from build123d import *

# Parameters (mm, degrees)
BOSS_EXTRUDE1_DEPTH = 4
SKETCH2_R           = 2.4
CUT_EXTRUDE1_DEPTH  = 12.510864433
SKETCH3_R           = 3.1
CUT_EXTRUDE2_DEPTH  = 1


with BuildPart() as part:
    # Sketch1 → Boss-Extrude1 (new, symmetric)
    with BuildSketch(Plane(origin=(0, 0, 0), x_dir=(1, 0, 0), z_dir=(0, 1, 0))):
        with BuildLine():
            Line((-4, 3.5), (4, 3.5))
            ThreePointArc((4, 3.5), (7.5, 0), (4, -3.5))
            Line((4, -3.5), (-4, -3.5))
            ThreePointArc((-4, -3.5), (-7.5, 0), (-4, 3.5))
        make_face()
    extrude(amount=BOSS_EXTRUDE1_DEPTH, both=True)

    # Sketch2 → Cut-Extrude1 (cut, through all)
    with BuildSketch(Plane(origin=(0, 4, 0), x_dir=(1, 0, 0), z_dir=(0, 1, 0))):
        with Locations(Location((4, 0, 0), (0, 0, 270))):
            Circle(SKETCH2_R)
        with BuildLine():
            Line((-4.84, -2.177705214), (-4.84, -1.24))
            ThreePointArc((-4.84, -1.24), (-4.957157288, -0.957157288), (-5.24, -0.84))
            Line((-5.24, -0.84), (-6.177705214, -0.84))
            ThreePointArc((-6.177705214, -0.84), (-6.235940121, -0.821293884), (-6.27238805, -0.772173913))
            ThreePointArc((-6.27238805, -0.772173913), (-6.4, 0), (-6.27238805, 0.772173913))
            ThreePointArc((-6.27238805, 0.772173913), (-6.235940121, 0.821293884), (-6.177705214, 0.84))
            Line((-6.177705214, 0.84), (-5.24, 0.84))
            ThreePointArc((-5.24, 0.84), (-4.957157288, 0.957157288), (-4.84, 1.24))
            Line((-4.84, 1.24), (-4.84, 2.177705214))
            ThreePointArc((-4.84, 2.177705214), (-4.821293884, 2.235940121), (-4.772173913, 2.27238805))
            ThreePointArc((-4.772173913, 2.27238805), (-4, 2.4), (-3.227826087, 2.27238805))
            ThreePointArc((-3.227826087, 2.27238805), (-3.178706116, 2.235940121), (-3.16, 2.177705214))
            Line((-3.16, 2.177705214), (-3.16, 1.24))
            ThreePointArc((-3.16, 1.24), (-3.042842712, 0.957157288), (-2.76, 0.84))
            Line((-2.76, 0.84), (-1.822294786, 0.84))
            Line((-1.822294786, 0.84), (-0.602294892, 0.84))
            ThreePointArc((-0.602294892, 0.84), (-0.767197546, 1.341263694), (-1.005585937, 1.812038747))
            ThreePointArc((-1.005585937, 1.812038747), (-1.042652048, 2.255086643), (-0.7121875, 2.552506408))
            ThreePointArc((-0.7121875, 2.552506408), (0, 2.65), (0.7121875, 2.552506408))
            ThreePointArc((0.7121875, 2.552506408), (1.042652048, 2.255086643), (1.005585937, 1.812038747))
            ThreePointArc((1.005585937, 1.812038747), (0.5, 0), (1.005585938, -1.812038747))
            ThreePointArc((1.005585938, -1.812038747), (1.042652048, -2.255086643), (0.7121875, -2.552506408))
            ThreePointArc((0.7121875, -2.552506408), (0, -2.65), (-0.7121875, -2.552506408))
            ThreePointArc((-0.7121875, -2.552506408), (-1.042652048, -2.255086643), (-1.005585937, -1.812038747))
            ThreePointArc((-1.005585937, -1.812038747), (-0.767197546, -1.341263694), (-0.602294892, -0.84))
            Line((-0.602294892, -0.84), (-1.822294786, -0.84))
            Line((-1.822294786, -0.84), (-2.76, -0.84))
            ThreePointArc((-2.76, -0.84), (-3.042842712, -0.957157288), (-3.16, -1.24))
            Line((-3.16, -1.24), (-3.16, -2.177705214))
            ThreePointArc((-3.16, -2.177705214), (-3.178706116, -2.235940121), (-3.227826087, -2.27238805))
            ThreePointArc((-3.227826087, -2.27238805), (-4, -2.4), (-4.772173913, -2.27238805))
            ThreePointArc((-4.772173913, -2.27238805), (-4.821293884, -2.235940121), (-4.84, -2.177705214))
        make_face()
    extrude(amount=-CUT_EXTRUDE1_DEPTH, mode=Mode.SUBTRACT)

    # Sketch3 → Cut-Extrude2 (cut)
    with BuildSketch(Plane(origin=(0, 4, 0), x_dir=(1, 0, 0), z_dir=(0, 1, 0))):
        with Locations(Location((4, 0, 0), (0, 0, 270))):
            Circle(SKETCH3_R)
    cut_extrude2 = extrude(amount=-CUT_EXTRUDE2_DEPTH, mode=Mode.SUBTRACT)

    # Mirror1: Cut-Extrude2 across plane
    add(cut_extrude2.mirror(Plane.ZX), mode=Mode.SUBTRACT)


solid = part.part
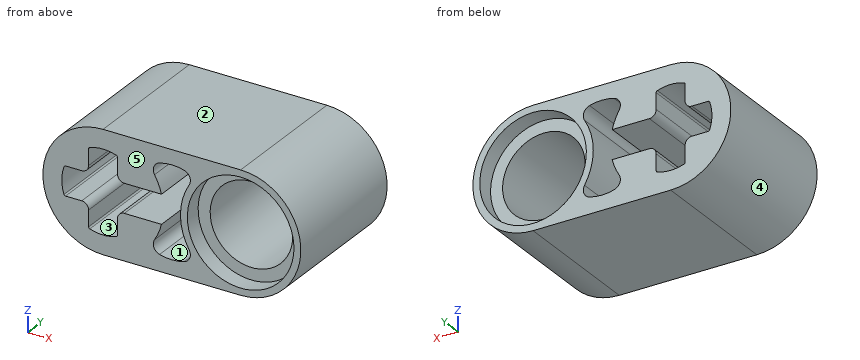
Could you check a few things on this model? Use its own coordinates, in mm. Face numbers are marked on the shaded views. A direction names the side the tool comes from. Round coordinates to 2 decimals unless told otherwise and drop trailing zeros. Loops run counter-clockwise (first coordinate to the right, second up) from the corner with the lowest first, then second, coordinate; pieces in that order, holes last. Notation, with made-up numbers: (72.25, -14.5) - (82.25, -14.5) arc R20 ccw to (82.25, -4.5) - close; hole circle Ø7 at (64.5, 34.25). An arc over 180 degrees is marked (long way). Write item = value, one per line.
1) Imagine slicing it at B-B (x = 5.5). Please give me the cut outline in (y, z), and give its area (3 significant figures).
Computed:
outline = (-4, -3.16) - (4, -3.16) - (4, -2.71) - (3, -2.71) - (3, -1.87) - (-3, -1.87) - (-3, -2.71) - (-4, -2.71) - close; (-4, 2.71) - (-3, 2.71) - (-3, 1.87) - (3, 1.87) - (3, 2.71) - (4, 2.71) - (4, 3.16) - (-4, 3.16) - close
area = 17.3 mm2
2) On a 3-axis mill with a long thin cutter (end or side, diameter ignored), from which of +Z, -Z, +X, -X, +Y, -Y can I reach the whole of each face in a straight line? I mean the marked faces 1 and 2. Say none if no direction works.
Computed:
face_1 = +Y, -Y
face_2 = +Z, +X, -X, +Y, -Y
3) Imagine slicing it at A-A (z = -2). Please give me the cut outline in (x, y), and give its area (3 significant figures).
Computed:
outline = (-6.87, -4) - (-4.84, -4) - (-4.84, 4) - (-6.87, 4) - close; (-3.16, -4) - (-1.07, -4) - (-1.07, 4) - (-3.16, 4) - close; (1.07, -4) - (1.63, -4) - (1.63, -3) - (2.67, -3) - (2.67, 3) - (1.63, 3) - (1.63, 4) - (1.07, 4) - close; (5.33, -3) - (6.37, -3) - (6.37, -4) - (6.87, -4) - (6.87, 4) - (6.37, 4) - (6.37, 3) - (5.33, 3) - close
area = 54.0 mm2
4) If we mould it in two halves opening along Z, with no side actions, what happens to the marked faces 3, 4 and 5? For each: pulls with the +Z half, pulls with the -Z half, needs draft (parallel to the pull), parting line crosses it, or undercut.
Computed:
face_3 = undercut
face_4 = parting line crosses it
face_5 = needs draft
5) I need wall thicknesses on line 1 along Y through (x, z) = (6.75, 0.25); line 2 along Z through (x, y) = (-2.25, 1.25); line 3 along Z through (x, y) = (-1, 0.5). Which ranges of each line are inside material? Lowest first, please. Write a range as from..to.
Computed:
line_1 = -3..3
line_2 = -3.5..-0.84, 0.84..3.5
line_3 = -3.5..-2.34, -1.8..-0.84, 0.84..1.8, 2.34..3.5
6) I'm going to push flat-ended pins straight in: P1, Ø0.5, axis at x = -5.5, y = 0.5, coming from the -Z side; P2, Ø1, axis at y = 1.5, z = 1.5, coming from the -X side; P3, Ø1.5, axis at y = 1.5, z = 2.5, coming from the -X side. Where does each tip first touch, or does it pass through?
Computed:
P1 = -3.27
P2 = -7.35
P3 = -7.03
7) Imagine slicing it at C-C (y = -0.5). Give the number of separate pieces and of enclosed holes in the cut face, and give its area (3 significant figures).
Computed:
separate_pieces = 1
enclosed_holes = 2
area = 53.4 mm2
8) Imagine slicing it at D-D (x = 1.25). Please give me the cut outline in (y, z), and give its area (3 significant figures).
Computed:
outline = (-4, -3.5) - (4, -3.5) - (4, -1.43) - (3, -1.43) - (3, 1.43) - (4, 1.43) - (4, 3.5) - (-4, 3.5) - (-4, 1.43) - (-3, 1.43) - (-3, -1.43) - (-4, -1.43) - close
area = 50.3 mm2
